from build123d import *

# Parameters (mm, degrees)
SKETCH1_W                      = 80
SKETCH1_H                      = 50
BOSS_EXTRUDE1_DEPTH            = 10
SKETCH2_R                      = 5
CUT_EXTRUDE1_DEPTH             = 49.218253805
M3_CLEARANCE_HOLE1_D           = 3.4
M3_CLEARANCE_HOLE1_CSINK_D     = 3.45
M3_CLEARANCE_HOLE1_CSINK_ANGLE = 90


with BuildPart() as part:
    # Sketch1 → Boss-Extrude1 (new body)
    with BuildSketch(Plane(origin=(0, 0, 0), x_dir=(1, 0, 0), z_dir=(0, 1, 0))):
        Rectangle(SKETCH1_W, SKETCH1_H)
    extrude(amount=BOSS_EXTRUDE1_DEPTH)

    # Sketch2 → Cut-Extrude1 (cut, through all)
    with BuildSketch(Plane(origin=(0, 10, 0), x_dir=(1, 0, 0), z_dir=(0, 1, 0))):
        with Locations(Location((0, 0, 0), (0, 0, 270))):
            Circle(SKETCH2_R)
    extrude(amount=-CUT_EXTRUDE1_DEPTH, mode=Mode.SUBTRACT)

    # M3 Clearance Hole1 (through all)
    with Locations(Plane(origin=(0, 10, 0), x_dir=(1, 0, 0), z_dir=(0, 1, 0))):
        with Locations((-34, 19), (34, 19), (-34, -19), (34, -19)):
            CounterSinkHole(M3_CLEARANCE_HOLE1_D / 2, M3_CLEARANCE_HOLE1_CSINK_D / 2, counter_sink_angle=M3_CLEARANCE_HOLE1_CSINK_ANGLE)


solid = part.part
Source: CAD feature listing. Evaluate the final solid. Frame: model axes, mm. Round coordinates to 2 decimals unless told otherwise and drop trailing zeros. Loops run counter-clockwise (first coordinate to the right, second up) from the corner with the lowest first, then second, coordinate; pieces in that order, holes last. Notation, with made-up numbers: (66.5, 8.25) -> (110.5, 8.25) arc R25 cw to (110.5, 37.25) -> close; hole circle Ø2 at (-39.5, 13). An arc over 180 degrees is marked (long way). Answer as a JSON object with one key per item and string values. Group by question number.
Q1. Mould query, pull axis X, two halves, no side actions, for faces 1 (the flat face through (40, 5, 0)), 2 (the cylindrical face through (32.38, 4.92, 18.49)), 3 (the flat face through (-1, 10, -6)). Classes: pulls with the +X half, pulls with the -X half, needs draft (parallel to the pull), parting line crosses it, or undercut.
Q2. Contact query for a flat-ended pin moving along its axis: P1, Ø4, axis at x = 34, z = -19, coming from the +Y side. Output: stop coordinate, or through.
Q3. Section query D-D (z = -3). Output: boundary loops of the cut face in (x, y).
Q4. Ray query, line 1 (X direction, y = 4.25, z = 19); line 2 (Z direction, x = 34, y = 4.5); line 3 (X direction, y = 6.25, z = -18.5). Return the intervals inside material, ascending. Write a range as from..to.
Q5. Section query B-B (x = 34). Output: boundary loops of the cut face in (y, z) (3 decimals), plus the area to 3 significant figures.
Q6. Section query A-A (z = 19). Output: boundary loops of the cut face in (x, y) (3 decimals), plus the area to 3 significant figures.
Q7. Section query C-C (y = 5.25). Output: boundary loops of the cut face in (x, z).
Completed:
{
 "1": {"face 1": "pulls with the +X half", "face 2": "undercut", "face 3": "needs draft"},
 "2": {"P1": "y = 10"},
 "3": {"outline": "(-40, 0) -> (-4, 0) -> (-4, 10) -> (-40, 10) -> close; (4, 0) -> (40, 0) -> (40, 10) -> (4, 10) -> close"},
 "4": {"line 1": "-40..-35.7, -32.3..32.3, 35.7..40", "line 2": "-25..-20.7, -17.3..17.3, 20.7..25", "line 3": "-40..-35.62, -32.38..32.38, 35.62..40"},
 "5": {"outline": "(0, -25) -> (10, -25) -> (10, -20.725) -> (9.975, -20.7) -> (0, -20.7) -> close; (0, -17.3) -> (9.975, -17.3) -> (10, -17.275) -> (10, 17.275) -> (9.975, 17.3) -> (0, 17.3) -> close; (0, 20.7) -> (9.975, 20.7) -> (10, 20.725) -> (10, 25) -> (0, 25) -> close", "area": "432 mm²"},
 "6": {"outline": "(-40, 0) -> (-35.7, 0) -> (-35.7, 9.975) -> (-35.725, 10) -> (-40, 10) -> close; (-32.3, 0) -> (32.3, 0) -> (32.3, 9.975) -> (32.275, 10) -> (-32.275, 10) -> (-32.3, 9.975) -> close; (35.7, 0) -> (40, 0) -> (40, 10) -> (35.725, 10) -> (35.7, 9.975) -> close", "area": "732 mm²"},
 "7": {"outline": "(-40, -25) -> (40, -25) -> (40, 25) -> (-40, 25) -> close; hole circle Ø3.4 at (-34, -19); hole circle Ø3.4 at (-34, 19); hole circle Ø10 at (0, 0); hole circle Ø3.4 at (34, -19); hole circle Ø3.4 at (34, 19)"}
}
